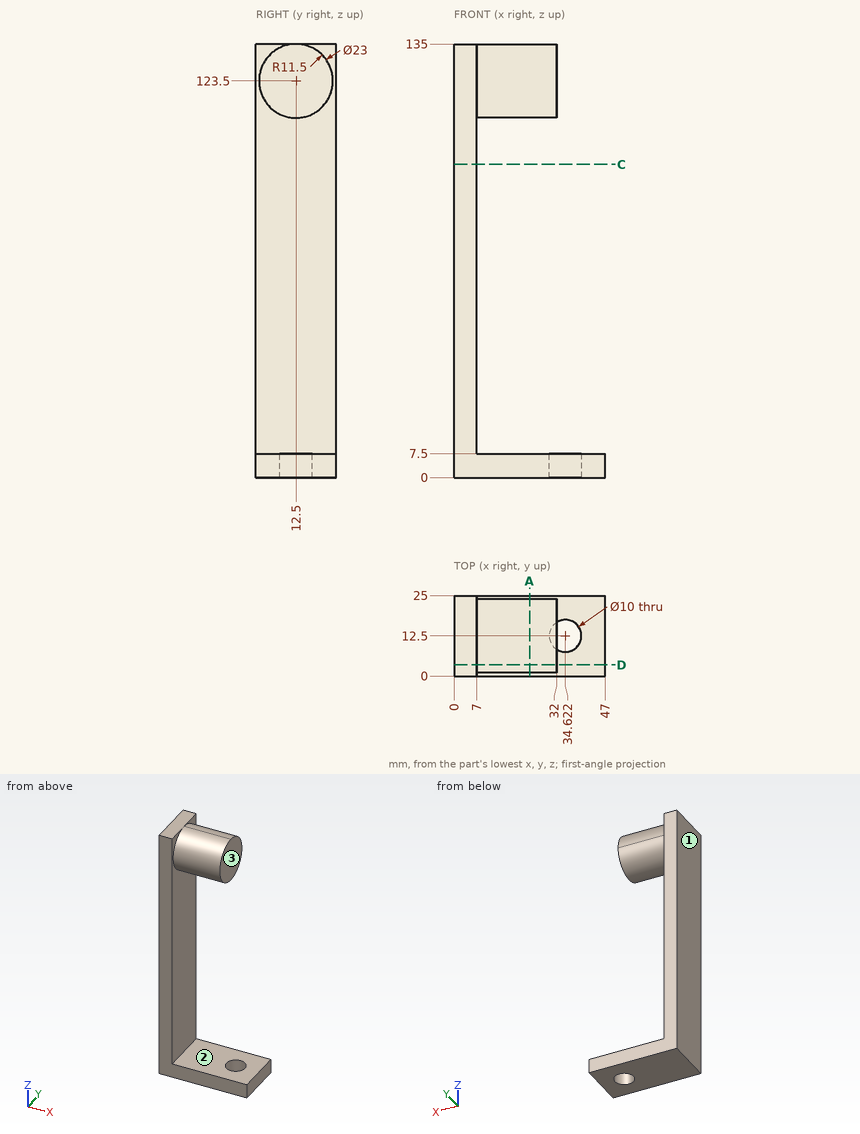
Input: dimensioned drawing with shaded views. Units: mm. Origin: part minimum x, y, z. A direction names the side the tool comes from. Coordinates: 2 decimals unless noted, no trailing zeros. Order: outer loops, then holes, each group sorted by start corner. A loop starts at its lowest first (then second) coordinate and runs counter-clockwise, first axis right, second up. Notation, with made-up numbers: (78, 61) - (84, 61) arc R10 cw to (84, 65) - close; hole circle Ø1 at (5, -2.5). An arc over 180 degrees is marked (long way). Put each result on its own line as item: value.
1. Cut plane D-D on y = 3.5. Return the cut outline in (x, z).
Report:
outline: (0, 0) - (47, 0) - (47, 7.5) - (7, 7.5) - (7, 116.34) - (32, 116.34) - (32, 130.66) - (7, 130.66) - (7, 135) - (0, 135) - close
2. Cut plane C-C on z = 97.5. Return the cut outline in (x, y).
Report:
outline: (0, 0) - (7, 0) - (7, 25) - (0, 25) - close
3. Reachability of the marked faces 1, 2 and 3 from +Z, -Z, +X, -X, +Y, -Y: full face, straight path, thin tool, end or side. Return the list, or none.
Report:
face 1: +Z, -Z, -X, +Y, -Y
face 2: +X, +Y, -Y
face 3: +Z, +X, +Y, -Y
4. Line query: line 1 along Z through (x, y) = (32.5, 5.5); line 2 along Z through (x, y) = (25.5, 12.5); line 3 along Z through (x, y) = (17, 14.25). Output: solid intervals per line, ascending.
Report:
line 1: z = 0 to 7.5
line 2: z = 0 to 7.5, 112 to 135
line 3: z = 0 to 7.5, 112.13 to 134.87
5. Cut plane A-A on x = 23.5. Return the cut outline in (y, z).
Report:
outline: (0, 0) - (25, 0) - (25, 7.5) - (0, 7.5) - close; circle Ø23 at (12.5, 123.5)
6. Contact query for flat-ended pins moving along their axis: pin 1 Ø1 at (x, y) = (28, 9) entering from +Z; pin 2 Ø8 at (y, z) = (13, 96) entering from +X; pin 3 Ø3 at (x, y) = (37, 16.5) entering from +Z. Output: stop coordinate, or through.
Report:
pin 1: stops at z = 134.6
pin 2: stops at x = 7
pin 3: stops at z = 7.5
